Read the model definition and answer for the solid it produces. Units are mm, in the model's axes. A direction names the side the tool comes from. Give positions to 0.01 mm unless a question says otherwise; leave off trailing zeros. Order: outer loops, then holes, each group sorted by start corner. A loop starts at its lowest first (then second) coordinate and runs counter-clockwise, first axis right, second up. Notation, with made-up numbers: (43, 78.5) - (77, 78.5) arc R23 cw to (77, 107.5) - close; hole circle Ø7 at (13, -14). An arc over 180 degrees is marked (long way). Use a Markdown table: item, result. Add a question column.
1. A cutting plane is placed at B-B on y = 191. Determine the outline of the cut face in (x, z).
2. A cutting plane is placed at A-A on z = 4. Determine the outline of the cut face in (x, y), and give its area (3 significant figures).
3. A cutting plane is placed at C-C on x = 13.5. Determine the outline of the cut face in (y, z).
4. Consider L1, parallel to X at y = 255, z = 3; L2, parallel to X at y = 293.5, z = 9; L3, parallel to Y at x = -6, z = 7.25. Determine where each line is inside the solid, lowest interval first.
5. Flat-ended cylindrical pins translate along their axes: P1, Ø6, axis at x = -16.5, z = 6, coming from the -Y side; P2, Ø3, axis at y = 281.5, z = 2, coming from the +X side; P3, Ø1, axis at x = 9.5, z = 2, coming from the -Y side. Find the tip coordinate at first contact, or state that the pin passes through.
6. Which of the six approach directions +Z, -Z, +X, -X, +Y, -Y give full straight-line access (tool end or side, diameter ignored) to faces 1 (the flat face through (10, 210, 5)), 2 (the flat face through (-10, 210, 5)), 3 (the cylindrical face through (0, 328, 6)), 4 (the flat face through (0, 146, 8))?
```python
from build123d import *

# Parameters (mm, degrees)
SKETCH_W     = 20
SKETCH_H     = 128
PAD_DEPTH    = 11
PAD001_DEPTH = 11
SKETCH002_W  = 7.9
SKETCH002_H  = 8
PAD002_DEPTH = 8


with BuildPart() as part:
    # Sketch → Pad (new body)
    with BuildSketch(Plane.XY):
        with Locations((0, 214)):
            Rectangle(SKETCH_W, SKETCH_H)
    extrude(amount=PAD_DEPTH)

    # Sketch001 (on Face6 of Pad) → Pad001 (join)
    with BuildSketch(Plane.XY.offset(11)):
        with BuildLine():
            ThreePointArc((27.5, 317.047375), (0, 328), (-27.5, 317.047375))
            Line((-27.5, 317.047375), (-27.5, 298.047375))
            ThreePointArc((-27.5, 298.047375), (0, 270.547415), (27.5, 298.047375))
            Line((27.5, 317.047375), (27.5, 298.047375))
        make_face()
    extrude(amount=-PAD001_DEPTH)

    # Sketch002 (on Face5 of Pad001) → Pad002 (join)
    with BuildSketch(Plane.XZ.offset(-150)):
        with Locations((0, 4)):
            Rectangle(SKETCH002_W, SKETCH002_H)
    extrude(amount=PAD002_DEPTH)


solid = part.part
```
Output values:
| question | item | result |
|---|---|---|
| 1 | outline | (-10, 0) - (10, 0) - (10, 11) - (-10, 11) - close |
| 2 | outline | (-27.5, 298.05) arc R27.5 ccw to (-10, 272.43) - (-10, 150) - (-3.95, 150) - (-3.95, 142) - (3.95, 142) - (3.95, 150) - (10, 150) - (10, 272.43) arc R27.5 ccw to (27.5, 298.05) - (27.5, 317.05) arc R40 ccw to (-27.5, 317.05) - close |
| 2 | area | 5,130 mm² |
| 3 | outline | (274.09, 0) - (325.65, 0) - (325.65, 11) - (274.09, 11) - close |
| 4 | L1 | -10 to 10 |
| 4 | L2 | -27.12 to 27.12 |
| 4 | L3 | 150 to 327.55 |
| 5 | P1 | y = 274.09 |
| 5 | P2 | x = 23.02 |
| 5 | P3 | y = 150 |
| 6 | face 1 | +Z, -Z, +X, -Y |
| 6 | face 2 | +Z, -Z, -X, -Y |
| 6 | face 3 | +Z, -Z, +Y |
| 6 | face 4 | +Z, +X, -X, -Y |
